Drawing for the job (mm, zero at the part's lowest x, y, z). Give positions to 0.01 mm unless a question says otherwise; leave off trailing zeros. Write each loop counter-clockwise with the first axis right and the second up, starting at its lowest first coordinate (ties: lowest second). Pieces come first, ordered by that corner, then holes.
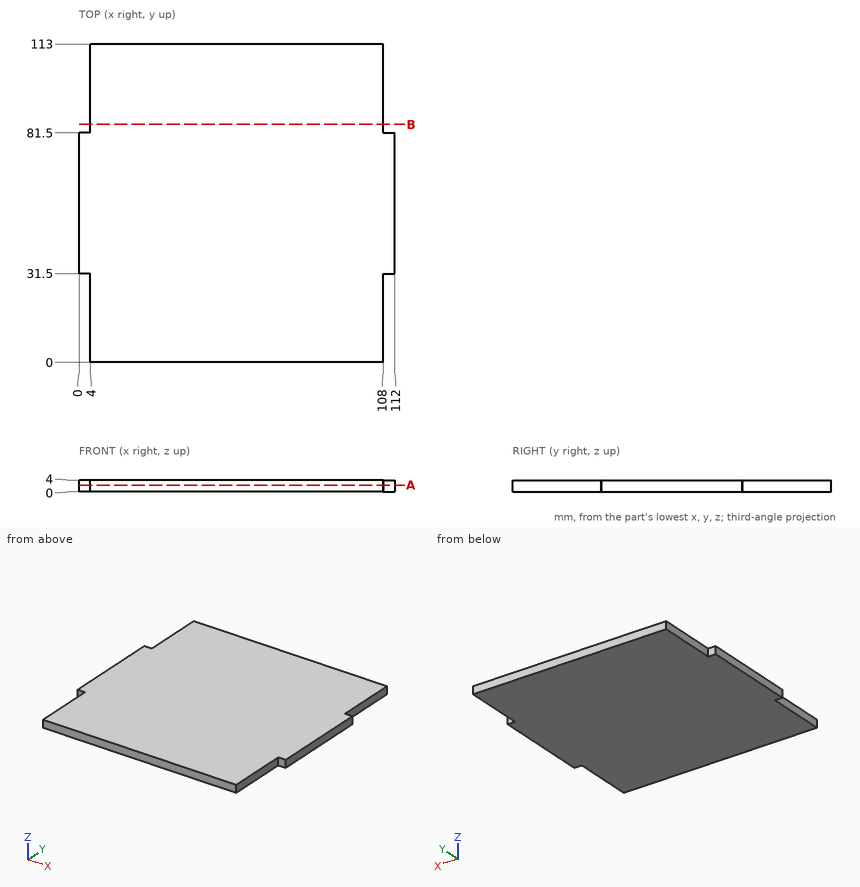
1. Probe probe 1 along X at (y, z) = (83.5, 1.35). List the from-to ranges inside material, lowest first.
Calculated:
probe 1: x = 4 to 108
2. Pin check, flat tips, straight feed: P1, Ø1.2, axis at y = 8.5, z = 1.5, coming from the -X side; P2, Ø1.5, axis at y = 87.5, z = 2.5, coming from the +X side; P3, Ø1.2, axis at x = 109, z = 1.5, coming from the -Y side. Stop position of each tip, or through.
Calculated:
P1: stops at x = 4
P2: stops at x = 108
P3: stops at y = 31.5
3. Slice it at A-A, the plane z = 2.35. Write the cut outline in (x, y), and give its area (3 significant figures).
Calculated:
outline: (0, 31.5) - (4, 31.5) - (4, 0) - (108, 0) - (108, 31.5) - (112, 31.5) - (112, 81.5) - (108, 81.5) - (108, 113) - (4, 113) - (4, 81.5) - (0, 81.5) - close
area: 12,200 mm2
4. Slice it at B-B, the plane y = 84.5. Write the cut outline in (x, z), and give its area (3 significant figures).
Calculated:
outline: (4, 0) - (108, 0) - (108, 4) - (4, 4) - close
area: 416 mm2
